Build history of the part. All positions in model axes, mm. Round coordinates to 2 decimals unless told otherwise and drop trailing zeros. Loops run counter-clockwise (first coordinate to the right, second up) from the corner with the lowest first, then second, coordinate; pieces in that order, holes last.
from build123d import *

# Parameters (mm, degrees)
SKETCH2_R           = 2.159
SKETCH2_W           = 88.9
SKETCH2_H           = 203.2
BOSS_EXTRUDE1_DEPTH = 3.175


with BuildPart() as part:
    # Sketch2 → Boss-Extrude1 (new body)
    with BuildSketch(Plane(origin=(0, 0, 0), x_dir=(1, 0, 0), z_dir=(0, 1, 0))):
        Polygon((0, 12.7), (0, 241.3), (12.7, 254), (114.3, 254), (127, 241.3), (127, 12.7), (114.3, 0), (12.7, 0), align=None)
        with Locations(Location((6.35, 165.1, 0), (0, 0, 270))):
            Circle(SKETCH2_R, mode=Mode.SUBTRACT)
        with Locations(Location((25.4, 247.65, 0), (0, 0, 270))):
            Circle(SKETCH2_R, mode=Mode.SUBTRACT)
        with Locations(Location((6.35, 203.2, 0), (0, 0, 270))):
            Circle(SKETCH2_R, mode=Mode.SUBTRACT)
        with Locations(Location((63.5, 247.65, 0), (0, 0, 270))):
            Circle(SKETCH2_R, mode=Mode.SUBTRACT)
        with Locations(Location((6.35, 127, 0), (0, 0, 270))):
            Circle(SKETCH2_R, mode=Mode.SUBTRACT)
        with Locations(Location((120.65, 127, 0), (0, 0, 270))):
            Circle(SKETCH2_R, mode=Mode.SUBTRACT)
        with Locations(Location((120.65, 165.1, 0), (0, 0, 270))):
            Circle(SKETCH2_R, mode=Mode.SUBTRACT)
        with Locations(Location((120.65, 203.2, 0), (0, 0, 270))):
            Circle(SKETCH2_R, mode=Mode.SUBTRACT)
        with Locations(Location((101.6, 247.65, 0), (0, 0, 270))):
            Circle(SKETCH2_R, mode=Mode.SUBTRACT)
        with Locations(Location((101.6, 6.35, 0), (0, 0, 270))):
            Circle(SKETCH2_R, mode=Mode.SUBTRACT)
        with Locations(Location((63.5, 6.35, 0), (0, 0, 270))):
            Circle(SKETCH2_R, mode=Mode.SUBTRACT)
        with Locations(Location((25.4, 6.35, 0), (0, 0, 270))):
            Circle(SKETCH2_R, mode=Mode.SUBTRACT)
        with Locations(Location((120.65, 50.8, 0), (0, 0, 270))):
            Circle(SKETCH2_R, mode=Mode.SUBTRACT)
        with Locations(Location((6.35, 50.8, 0), (0, 0, 270))):
            Circle(SKETCH2_R, mode=Mode.SUBTRACT)
        with Locations(Location((120.65, 88.9, 0), (0, 0, 270))):
            Circle(SKETCH2_R, mode=Mode.SUBTRACT)
        with Locations(Location((6.35, 88.9, 0), (0, 0, 270))):
            Circle(SKETCH2_R, mode=Mode.SUBTRACT)
        with Locations((63.5, 127)):
            Rectangle(SKETCH2_W, SKETCH2_H, mode=Mode.SUBTRACT)
    extrude(amount=BOSS_EXTRUDE1_DEPTH)


solid = part.part
(1) Slice it at A-A on z = -110.5. List the corners of the cut face in (x, y) (3 decimals).
Responses:
outline: (0, 0) - (19.05, 0) - (19.05, 3.175) - (0, 3.175) - close; (107.95, 0) - (127, 0) - (127, 3.175) - (107.95, 3.175) - close
(2) Slice it at C-C on y = 1. Count the separate pieces of the cut face and the enclosed holes in it, plus the area to 3 significant figures.
Responses:
separate pieces: 1
enclosed holes: 17
area: 13,600 mm2
(3) Probe line 1 (X direction, y = 1.15, z = -88.9); line 2 (Z direction, x = 94.5, y = 1.65); line 3 (X direction, y = 2.45, z = -110.5). List the from-to ranges inside material, lowest first.
Responses:
line 1: x = 0 to 4.19, 8.51 to 19.05, 107.95 to 118.49, 122.81 to 127
line 2: z = -254 to -228.6, -25.4 to 0
line 3: x = 0 to 19.05, 107.95 to 127
(4) Slice it at B-B on x = 54. List the corners of the cut face in (y, z) (3 decimals), plus the area to 3 significant figures.
Responses:
outline: (0, -254) - (3.175, -254) - (3.175, -228.6) - (0, -228.6) - close; (0, -25.4) - (3.175, -25.4) - (3.175, 0) - (0, 0) - close
area: 161 mm2
(5) Pin check, flat tips, straight feed: P1, Ø5, axis at x = 25.4, z = -6.35, coming from the +Y side (3 decimals); P2, Ø4, axis at x = 6.35, z = -165.1, coming from the +Y side. Stop position of each tip, or through.
Responses:
P1: stops at y = 3.175
P2: passes through
(6) Pull direction Z, two halves, no side cores. Call faces 1 (the face through (103.42, 1.57, -5.19)), 2 (the face through (8, 3.175, -129)), 3 (the face through (6.3, 1.6, -247.6)): +Z half, -Z half, draft (parallel to the pull), parting line (faces both ways), or undercut.
Responses:
face 1: undercut
face 2: draft
face 3: -Z half
